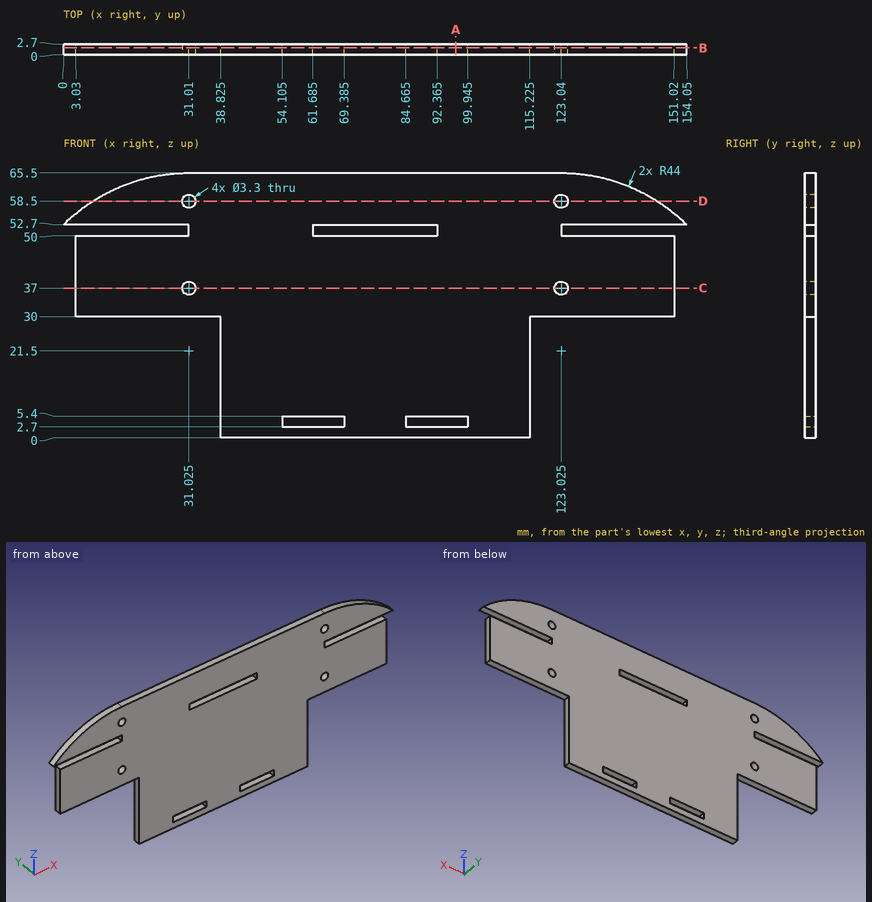
The figure shows three views and two pictorial views of one solid part (mm, origin at its lowest corner). Answer the questions. Give positions to 0.01 mm unless a question says otherwise; leave off trailing zeros. Write each loop counter-clockwise with the first axis right and the second up, starting at its lowest first coordinate (ties: lowest second). Pieces come first, ordered by that corner, then holes. Notation, with made-up numbers: (-10.5, 89.5) - (5.5, 89.5) arc R23 cw to (5.5, 118.5) - close; hole circle Ø6 at (-17.5, -29). An arc over 180 degrees is marked (long way). Return JSON: item names as keys, results as strings.
Q1. A cutting plane is placed at B-B, the plane y = 1.75. Count the separate pieces of the cut face and the enclosed holes in it.
Reply:
{"separate pieces": "1", "enclosed holes": "7"}
Q2. A cutting plane is placed at A-A, the plane x = 97. Determine the outline of the cut face in (y, z).
Reply:
{"outline": "(0, 0) - (2.7, 0) - (2.7, 2.7) - (0, 2.7) - close; (0, 5.4) - (2.7, 5.4) - (2.7, 65.5) - (0, 65.5) - close"}
Q3. Given P1, Ø1, axis at x = 138.5, y = 1, coming from the -Z side; P2, Ø1.4, axis at y = 1.5, z = 20, coming from the +X side (3 decimals); P3, Ø1.4, axis at y = 1.5, z = 4.5, coming from the -X side (3 decimals); P4, Ø10, axis at x = 19.5, z = 22, coming from the -Y side, each flat-ended and moving along its own axis, determine where each tip first touches the part or whether it passes through.
Reply:
{"P1": "z = 30", "P2": "x = 115.225", "P3": "x = 38.825", "P4": "through"}
Q4. A cutting plane is placed at D-D, the plane z = 58.5. Determine the outline of the cut face in (x, y) (1 decimal), and give its area (3 significant figures).
Reply:
{"outline": "(7.2, 0) - (29.4, 0) - (29.4, 2.7) - (7.2, 2.7) - close; (32.7, 0) - (121.4, 0) - (121.4, 2.7) - (32.7, 2.7) - close; (124.7, 0) - (146.8, 0) - (146.8, 2.7) - (124.7, 2.7) - close", "area": "359 mm²"}
Q5. Consider line 1 along Z through (x, y) = (86.5, 2.45); line 2 along X through (y, z) = (2.05, 37) (1 decimal); line 3 along Z through (x, y) = (80, 2.55). Determine where each line is inside the solid, lowest interval first. Write a range as [from, to].
Reply:
{"line 1": "[0, 2.7], [5.4, 50], [52.7, 65.5]", "line 2": "[3, 29.4], [32.7, 121.4], [124.7, 151]", "line 3": "[0, 50], [52.7, 65.5]"}
Q6. A cutting plane is placed at C-C, the plane z = 37. Determine the outline of the cut face in (x, y) (1 decimal), and give its area (3 significant figures).
Reply:
{"outline": "(3, 0) - (29.4, 0) - (29.4, 2.7) - (3, 2.7) - close; (32.7, 0) - (121.4, 0) - (121.4, 2.7) - (32.7, 2.7) - close; (124.7, 0) - (151, 0) - (151, 2.7) - (124.7, 2.7) - close", "area": "382 mm²"}
